from build123d import *

# Parameters (mm, degrees)
F1_DEPTH = 100
F3_START = -45
F3_DEPTH = 10
F4_R     = 4
F5_W     = 60
F5_H     = 8.6717781019
F6_DEPTH = 4
F7_R     = 3.99999


# Not quite as in the source:
# - a fillet or chamfer is up to 0.001 mm smaller than in the source, because OpenCascade refuses the exact size


with BuildPart() as f1:
    # F0 (on Right) → F1 (new body)
    with BuildSketch(Plane.YZ):
        Polygon((-5.0582498297, 30.4073218231), (-8.1640783709, 30.4073218231), (-15.2398989277, 4), (-24.5573845514, 4), (-23.4855877816, 8), (-26.5914163229, 8), (-28.7350098623, 0), (-13.2058671562, 0), align=None)
    extrude(amount=F1_DEPTH)

    # F2 (on face) → F3 (join)
    with BuildSketch(Plane(origin=(0, 0, 0), x_dir=(0, -1, 0), z_dir=(-1, 0, 0)).offset(F3_START)):
        Polygon((13.2058671562, 0), (6.7691872092, 24.0220165943), (-22.3890729249, 3.8824980147), (-22.3890729249, 0), align=None)
    extrude(amount=-F3_DEPTH)

    # F4 (call 1 of 6: OpenCascade refuses the feature's edges together)
    f4_edges = [f1.edges().sort_by_distance(p)[0] for p in [
        (0, -6.611164, 30.407322),
    ]]
    fillet(f4_edges, radius=F4_R)

    # F4#2 (call 2 of 6)
    f4_2_edges = [f1.edges().sort_by_distance(p)[0] for p in [
        (100, -6.611164, 30.407322),
    ]]
    fillet(f4_2_edges, radius=F4_R)

    # F4#3 (call 3 of 6)
    f4_3_edges = [f1.edges().sort_by_distance(p)[0] for p in [
        (100, -25.038502, 8),
    ]]
    fillet(f4_3_edges, radius=F4_R)

    # F4#4 (call 4 of 6)
    f4_4_edges = [f1.edges().sort_by_distance(p)[0] for p in [
        (0, -25.038502, 8),
    ]]
    fillet(f4_4_edges, radius=F4_R)

    # F4#5 (call 5 of 6)
    f4_5_edges = [f1.edges().sort_by_distance(p)[0] for p in [
        (50, 22.389073, 3.882498),
    ]]
    fillet(f4_5_edges, radius=F4_R)

    # F4#6 (call 6 of 6)
    f4_6_edges = [f1.edges().sort_by_distance(p)[0] for p in [
        (50, -6.769187, 24.022017),
        (45, -9.987527, 12.011008),
        (55, -9.987527, 12.011008),
    ]]
    fillet(f4_6_edges, radius=F4_R)

    # F5 (on face) → F6 (cut)
    with BuildSketch(Plane.XY.offset(8)):
        with Locations((50, -27.8214768326)):
            Rectangle(F5_W, F5_H)
    extrude(amount=-F6_DEPTH, mode=Mode.SUBTRACT)

    # F7 (radius 4 in the source; OpenCascade refuses exactly that, so slightly less here)
    f7_edges = [f1.edges().sort_by_distance(p)[0] for p in [
        (20, -25.038502, 8),
        (80, -25.038502, 8),
    ]]
    fillet(f7_edges, radius=F7_R)


solid = f1.part
Check sheet for the modelled part. Datum: model origin and axes. Units: mm. A direction names the side the tool comes from. Round coordinates to 2 decimals unless told otherwise and drop trailing zeros. Loops run counter-clockwise (first coordinate to the right, second up) from the corner with the lowest first, then second, coordinate; pieces in that order, holes last. Notation, with made-up numbers: (10.5, 15.25) -> (41.5, 15.25) arc R27 cw to (41.5, 32.25) -> close; hole circle Ø3 at (-30, -5). An arc over 180 degrees is marked (long way). Put each result on its own line as item: value. Start each with the question number.
1. Draft check along Y on faces 6 (the face through (90, -25, 8)), 7 (the face through (38.19, -9.19, 14.99)), 8 (the face through (89.86, -24.03, 5.97)). Enter one of: +Y half, -Y half, draft (parallel to the pull), parting line (faces both ways), or undercut.
2. Section check A-A (x = 85). Enter the section's corners in (y, z) (3 decimals).
3. Access from +Z, -Z, +X, -X, +Y, -Y to the whole of each face (thin tool, end or side, straight path). Record for faces 1 (the face through (10, -25, 8)), 2 (the face through (45, 3, 9)), 3 (the face through (1.203, -25.604, 6.859)), 4 (the face through (98.859, -25.604, 6.797)), 5 (the face through (81.203, -25.545, 6.859)).
4. Section check B-B (y = -21.5). Enter the section's corners in (x, z), plus the area to 3 significant figures.
5. Section check C-C (x = 37.5). Enter the section's corners in (y, z) (3 decimals).
6. Scan lines: probe 1 along Y at (x, z) = (13.5, 5); probe 2 along Z at (x, y) = (10.5, -19); probe 3 along X at (y, z) = (19, 6). Record each from-to range of solid material in increasing order.
7. Section check D-D (z = 28.5). Enter the section's corners in (x, y), plus the area to 3 significant figures.
8. Gauge pin test, flat ends, axial feed: pin 1 (4 mm diameter, centred on x = 30, z = 6, fed in from +Y); pin 2 (10 mm diameter, centred on x = 72.5, z = 20.5, fed in from +Y); pin 3 (1 mm diameter, centred on x = 56.5, z = 24, fed in from +Y). Record the tip position at first contact, or that the pin passes through.
Findings:
1. face 6: draft
1. face 7: +Y half
1. face 8: undercut
2. outline: (-28.735, 0) -> (-13.206, 0) -> (-5.058, 30.407) -> (-8.164, 30.407) -> (-15.24, 4) -> (-24.557, 4) -> (-23.486, 8) -> (-26.591, 8) -> close
3. face 1: +Z, +X, -X, -Y
3. face 2: -Z, -X, +Y
3. face 3: +Z, -X, -Y
3. face 4: +Z, +X, -Y
3. face 5: +Z, -Y
4. outline: (0, 0) -> (100, 0) -> (100, 4) -> (0, 4) -> close
4. area: 400 mm^2
5. outline: (-28.735, 0) -> (-13.206, 0) -> (-5.058, 30.407) -> (-8.164, 30.407) -> (-15.24, 4) -> (-27.663, 4) -> close
6. probe 1: y = -27.4 to -24.29, -14.97 to -11.87
6. probe 2: z = 0 to 4
6. probe 3: x = 45 to 55
7. outline: (0.59, -8.68) -> (99.41, -8.68) -> (99.41, -5.57) -> (0.59, -5.57) -> close
7. area: 307 mm^2
8. pin 1: stops at y = -11.06
8. pin 2: stops at y = -6.37
8. pin 3: stops at y = -5.61
